from build123d import *

# Parameters (mm, degrees)
SKETCH1_W            = 250
SKETCH1_H            = 80
BOSS_EXTRUDE1_DEPTH  = 10
BOSS_EXTRUDE2_DEPTH  = 10
SKETCH3_R            = 2
CUT_EXTRUDE1_DEPTH   = 266.725892604
FILLET1_R            = 2.5
FILLET1_OF_MIRROR1_R = 2.5
MIRROR3_DEPTH        = 10
MIRROR3_2_DEPTH      = 10
FILLET2_R            = 5


# Read off the part's stored shape, not the designer's step: Mirror3
with BuildPart() as part:
    # Sketch1 → Boss-Extrude1 (new body)
    with BuildSketch(Plane.XY):
        with Locations((125, 40)):
            Rectangle(SKETCH1_W, SKETCH1_H)
    extrude(amount=BOSS_EXTRUDE1_DEPTH)

    # Sketch2 → Boss-Extrude2 (add)
    with BuildSketch(Plane.XY.offset(10)):
        with BuildLine():
            Line((49.65, 80), (100.35, 80))
            Line((100.35, 80), (100.35, 87))
            ThreePointArc((100.35, 87), (99.617766953, 88.767766953), (97.85, 89.5))
            Line((97.85, 89.5), (52.15, 89.5))
            ThreePointArc((52.15, 89.5), (50.382233047, 88.767766953), (49.65, 87))
            Line((49.65, 87), (49.65, 80))
        make_face()
    boss_extrude2 = extrude(amount=-BOSS_EXTRUDE2_DEPTH)

    # Sketch3 → Cut-Extrude1 (cut, through all)
    with BuildSketch(Plane.XY.offset(10)):
        with Locations((49.65, 80)):
            Circle(SKETCH3_R)
        with Locations((100.35, 80)):
            Circle(SKETCH3_R)
        Polygon((55.65, 80), (72, 80), (72, 89.5), (78, 89.5), (78, 80), (94.35, 80), (94.35, 74), (55.65, 74), align=None)
    cut_extrude1 = extrude(amount=-CUT_EXTRUDE1_DEPTH, mode=Mode.SUBTRACT)

    # Fillet1
    fillet1_edges = [part.edges().sort_by_distance(p)[0] for p in [
        (49.65, 82, 5),
        (100.35, 82, 5),
        (55.65, 74, 5),
        (55.65, 80, 5),
        (72, 80, 5),
        (72, 89.5, 5),
        (78, 89.5, 5),
        (78, 80, 5),
        (94.35, 80, 5),
        (94.35, 74, 5),
    ]]
    fillet(fillet1_edges, radius=FILLET1_R)

    # Mirror1: Boss-Extrude2, Cut-Extrude1 across plane
    add(boss_extrude2.mirror(Plane.ZY.offset(-125)))
    add(cut_extrude1.mirror(Plane.ZY.offset(-125)), mode=Mode.SUBTRACT)

    # Fillet1 of Mirror1
    fillet1_of_mirror1_edges = [part.edges().sort_by_distance(p)[0] for p in [
        (200.35, 82, 5),
        (149.65, 82, 5),
        (194.35, 74, 5),
        (194.35, 80, 5),
        (178, 80, 5),
        (178, 89.5, 5),
        (172, 89.5, 5),
        (172, 80, 5),
        (155.65, 80, 5),
        (155.65, 74, 5),
    ]]
    fillet(fillet1_of_mirror1_edges, radius=FILLET1_OF_MIRROR1_R)

    # Mirror3 outline → Mirror3 (cut)
    with BuildSketch(Plane.XY):
        with BuildLine():
            Line((47.65, 0), (51.65, 0))
            ThreePointArc((51.65, 0), (49.65, 2), (47.65, 0))
        make_face()
        with BuildLine():
            ThreePointArc((202.35, 0), (200.35, 2), (198.35, 0))
            Line((198.35, 0), (202.35, 0))
        make_face()
        with BuildLine():
            ThreePointArc((151.65, 0), (149.65, 2), (147.65, 0))
            Line((147.65, 0), (151.65, 0))
        make_face()
        with BuildLine():
            ThreePointArc((102.35, 0), (100.35, 2), (98.35, 0))
            Line((98.35, 0), (102.35, 0))
        make_face()
        with BuildLine():
            ThreePointArc((55.65, 2.5), (56.382233047, 0.732233047), (58.15, 0))
            Line((58.15, 0), (91.85, 0))
            ThreePointArc((91.85, 0), (93.617766953, 0.732233047), (94.35, 2.5))
            Line((94.35, 2.5), (94.35, 3.5))
            ThreePointArc((94.35, 3.5), (93.617766953, 5.267766953), (91.85, 6))
            Line((91.85, 6), (58.15, 6))
            ThreePointArc((58.15, 6), (56.382233047, 5.267766953), (55.65, 3.5))
            Line((55.65, 3.5), (55.65, 2.5))
        make_face()
        with BuildLine():
            ThreePointArc((155.65, 2.5), (156.382233047, 0.732233047), (158.15, 0))
            Line((158.15, 0), (191.85, 0))
            ThreePointArc((191.85, 0), (193.617766953, 0.732233047), (194.35, 2.5))
            Line((194.35, 2.5), (194.35, 3.5))
            ThreePointArc((194.35, 3.5), (193.617766953, 5.267766953), (191.85, 6))
            Line((191.85, 6), (158.15, 6))
            ThreePointArc((158.15, 6), (156.382233047, 5.267766953), (155.65, 3.5))
            Line((155.65, 3.5), (155.65, 2.5))
        make_face()
    extrude(amount=MIRROR3_DEPTH, mode=Mode.SUBTRACT)

    # Mirror3 2 outline → Mirror3 2 (add)
    with BuildSketch(Plane.XY):
        with BuildLine():
            Line((169.5, 0), (151.65, 0))
            ThreePointArc((151.65, 0), (151.413834207, -0.942809042), (150.761111111, -1.662958839))
            ThreePointArc((150.761111111, -1.662958839), (149.945207241, -2.563146085), (149.65, -3.741657387))
            Line((149.65, -3.741657387), (149.65, -7))
            ThreePointArc((149.65, -7), (150.382233047, -8.767766953), (152.15, -9.5))
            Line((152.15, -9.5), (169.5, -9.5))
            ThreePointArc((169.5, -9.5), (171.267766953, -8.767766953), (172, -7))
            Line((172, -7), (172, -2.5))
            ThreePointArc((172, -2.5), (171.267766953, -0.732233047), (169.5, 0))
        make_face()
        with BuildLine():
            Line((49.65, -3.741657387), (49.65, -7))
            ThreePointArc((49.65, -7), (50.382233047, -8.767766953), (52.15, -9.5))
            Line((52.15, -9.5), (69.5, -9.5))
            ThreePointArc((69.5, -9.5), (71.267766953, -8.767766953), (72, -7))
            Line((72, -7), (72, -2.5))
            ThreePointArc((72, -2.5), (71.267766953, -0.732233047), (69.5, 0))
            Line((69.5, 0), (51.65, 0))
            ThreePointArc((51.65, 0), (51.413834207, -0.942809042), (50.761111111, -1.662958839))
            ThreePointArc((50.761111111, -1.662958839), (49.945207241, -2.563146085), (49.65, -3.741657387))
        make_face()
        with BuildLine():
            Line((98.35, 0), (80.5, 0))
            ThreePointArc((80.5, 0), (78.732233047, -0.732233047), (78, -2.5))
            Line((78, -2.5), (78, -7))
            ThreePointArc((78, -7), (78.732233047, -8.767766953), (80.5, -9.5))
            Line((80.5, -9.5), (97.85, -9.5))
            ThreePointArc((97.85, -9.5), (99.617766953, -8.767766953), (100.35, -7))
            Line((100.35, -7), (100.35, -3.741657387))
            ThreePointArc((100.35, -3.741657387), (100.054792759, -2.563146085), (99.238888889, -1.662958839))
            ThreePointArc((99.238888889, -1.662958839), (98.586165793, -0.942809042), (98.35, 0))
        make_face()
        with BuildLine():
            Line((198.35, 0), (180.5, 0))
            ThreePointArc((180.5, 0), (178.732233047, -0.732233047), (178, -2.5))
            Line((178, -2.5), (178, -7))
            ThreePointArc((178, -7), (178.732233047, -8.767766953), (180.5, -9.5))
            Line((180.5, -9.5), (197.85, -9.5))
            ThreePointArc((197.85, -9.5), (199.617766953, -8.767766953), (200.35, -7))
            Line((200.35, -7), (200.35, -3.741657387))
            ThreePointArc((200.35, -3.741657387), (200.054792759, -2.563146085), (199.238888889, -1.662958839))
            ThreePointArc((199.238888889, -1.662958839), (198.586165793, -0.942809042), (198.35, 0))
        make_face()
    extrude(amount=MIRROR3_2_DEPTH)

    # Fillet2
    fillet2_edges = [part.edges().sort_by_distance(p)[0] for p in [
        (202.35, 80, 5),
        (147.65, 80, 5),
        (202.35, 0, 5),
        (147.65, 0, 5),
        (47.65, 80, 5),
        (47.65, 0, 5),
        (102.35, 0, 5),
        (102.35, 80, 5),
        (0, 80, 5),
        (250, 80, 5),
        (250, 0, 5),
        (0, 0, 5),
    ]]
    fillet(fillet2_edges, radius=FILLET2_R)


solid = part.part
Build history of the part. All positions in model axes, mm. A direction names the side the tool comes from. Coordinates: 2 decimals unless noted, no trailing zeros. Order: outer loops, then holes, each group sorted by start corner. A loop starts at its lowest first (then second) coordinate and runs counter-clockwise, first axis right, second up. Notation, with made-up numbers: (18, -31) - (56, -31) arc R21 cw to (56, -3) - close; hole circle Ø4 at (-10.5, 12.25). An arc over 180 degrees is marked (long way). Put each result on its own line as item: value.
1. Saw through at A-A (x = 23). Write the cut outline in (y, z), and give its area (3 significant figures).
Answer sheet:
outline: (0, 0) - (80, 0) - (80, 10) - (0, 10) - close
area: 800 mm^2
2. Drop flat-ended pins along their axis: P1, Ø1.5, axis at x = 111.5, y = 14.5, coming from the -Z side; P2, Ø0.8, axis at y = 77, z = 4, coming from the -X side; P3, Ø3.5, axis at x = 100.35, y = 80, coming from the -Z side; P4, Ø5, axis at y = 84.5, z = 2.5, coming from the +X side. Give the stop position or say it passes through.
Answer sheet:
P1: stops at z = 0
P2: stops at x = 0.26
P3: passes through
P4: stops at x = 200.35
3. Probe line 1 along X through (y, z) = (-5, 5.25); line 2 along Y through (x, z) = (85, 5.75); line 3 along Y through (x, z) = (238, 8.5). List the from-to ranges inside material, lowest first. Write a range as [from, to].
Answer sheet:
line 1: x = [49.65, 72], [78, 100.35], [149.65, 172], [178, 200.35]
line 2: y = [-9.5, 0], [6, 74], [80, 89.5]
line 3: y = [0, 80]
4. Pull direction X, two halves, no side cores. Call faces 5 (the face through (86, 80, 5)), 6 (the face through (123, 41, 0)), 7 (the face through (250, 40, 5)), 8 (the face through (164, 0, 5)): pulls with the +X half, pulls with the -X half, needs draft (parallel to the pull), parting line crosses it, or undercut.
Answer sheet:
face 5: undercut
face 6: needs draft
face 7: pulls with the +X half
face 8: undercut
5. Tool access for faces 1 (the face through (225, 0, 5)), 2 (the face through (178, 85, 5)), 3 (the face through (186, 80, 5)), 4 (the face through (178, -5, 5)): list every direction of +Z, -Z, +X, -X, +Y, -Y with a clear straight run to the whole face (end or side of a thin tool).
Answer sheet:
face 1: +Z, -Z, +X, -Y
face 2: +Z, -Z, +Y
face 3: +Z, -Z
face 4: +Z, -Z, -Y
